Autodesk Inventor part; units mm, degrees
ref_plane "YZ Plane" through (0, 0, 0) normal (1, 0, 0) x (0, 1, 0)
ref_plane "XZ Plane" through (0, 0, 0) normal (0, 1, 0) x (-1, 0, 0)
ref_plane "XY Plane" through (0, 0, 0) normal (0, 0, 1) x (1, 0, 0)
sketch "Sketch1" plane through (0, 0, 0) normal (0, 0, 1) x (1, 0, 0)
  line L0 (0, 9) -> (3.5, 9)
  line L1 (3.5, 9) -> (3.5, 6)
  line L2 (3.5, 6) -> (5, 6)
  line L3 (5, 6) -> (5, 3)
  line L4 (5, 3) -> (3.5, 3)
  line L5 (3.5, 3) -> (3.5, 0)
  line L6 (3.5, 0) -> (0, 0)
  line L7 (0, 0) -> (0, 9)
  dimension "d0" = 3
  dimension "d1" = 3
  dimension "d2" = 3
  dimension "d3" = 7
  dimension "d4" = 10
revolve "Revolution1" add sketch "Sketch1" angle 360 about axis through (0, 0, 0) along (0, 1, 0)
sketch "Sketch2" plane through (0, 9, 0) normal (0, 1, 0) x (1, 0, 0)
  circle A0 centre (0, 0) radius 3.5
hole "Hole1" at (0, 9, 0) direction (0, -1, 0) diameter 3 depth 9 countersink diameter 6 countersink angle 90
properties part number "26a"
Model file for the job. Use its own axes, mm. A direction names the side the tool comes from. Round coordinates to 2 decimals unless told otherwise and drop trailing zeros. Write each loop counter-clockwise with the first axis right and the second up, starting at its lowest first coordinate (ties: lowest second). Pieces come first, ordered by that corner, then holes. Notation, with made-up numbers: M 86,11.25 L 101,11.25 A9 cw 101,24.25 Z; hole C 81,-26 d7. An arc over 180 degrees is marked long. Put each result on its own line as item: value.
Item 1: Cut at D-D (z = -3.25). List the corners of the cut face in (x, y).
Responses:
outline: M -3.8,3 L -1.3,3 L -1.3,0 L 1.3,0 L 1.3,3 L 3.8,3 L 3.8,6 L 1.3,6 L 1.3,9 L -1.3,9 L -1.3,6 L -3.8,6 Z
Item 2: Cut at B-B (z = 0). List the corners of the cut face in (x, y), and give its area (4 significant figures).
Responses:
outline: M -5,3 L -3.5,3 L -3.5,0 L -1.5,0 L -1.5,7.5 L -3,9 L -3.5,9 L -3.5,6 L -5,6 Z; M 1.5,0 L 3.5,0 L 3.5,3 L 5,3 L 5,6 L 3.5,6 L 3.5,9 L 3,9 L 1.5,7.5 Z
area: 42.75 mm²
Item 3: Flat gauge pin, fed straight in: P1, Ø1.5, axis at y = 2.5, z = 3, coming from the -X side. Where does the tip first touch, or does it go through?
Responses:
P1: x = -4.36
Item 4: Cut at A-A (x = 0). List the corners of the cut face in (y, z), and give its area (4 significant figures).
Responses:
outline: M 0,-3.5 L 3,-3.5 L 3,-5 L 6,-5 L 6,-3.5 L 9,-3.5 L 9,-3 L 7.5,-1.5 L 0,-1.5 Z; M 0,1.5 L 7.5,1.5 L 9,3 L 9,3.5 L 6,3.5 L 6,5 L 3,5 L 3,3.5 L 0,3.5 Z
area: 42.75 mm²
Item 5: Tool access for faces 1 (the cylindrical face through (3.233, 1.479, -1.341)), 2 (the flat face through (2.2, 6, 3.3)), 3 (the flat face through (3, 9, -1)): list every direction of +Z, -Z, +X, -X, +Y, -Y with a clear straight run to the whole face (end or side of a thin tool).
Responses:
face 1: -Y
face 2: +Y
face 3: +Z, -Z, +X, -X, +Y
Item 6: Cut at C-C (y = 2.5). List the corners of the cut face in (x, z).
Responses:
outline: C 0,0 d7; hole C 0,0 d3
Item 7: Probe L1, parallel to Z at x = 0, y = 2.5; L2, parallel to Z at x = 0, y = 4.5. List the from-to ranges inside material, lowest first. Write a range as from..to.
Responses:
L1: -3.5..-1.5, 1.5..3.5
L2: -5..-1.5, 1.5..5
Item 8: Mould opens along Z. For faces 4 (the cylindrical face through (-0.07, 3.7, -1.5)), 5 (the flat face through (0, 0, 2)), 6 (the cylindrical face through (-1.08, 4.48, -4.88)) say: +Z half, -Z half, draft (parallel to the pull), parting line (faces both ways), or undercut.
Responses:
face 4: undercut
face 5: draft
face 6: parting line
